Verification items for the finished model (mm, model axes). Coordinates: 2 decimals unless noted, no trailing zeros. Order: outer loops, then holes, each group sorted by start corner. A loop starts at its lowest first (then second) coordinate and runs counter-clockwise, first axis right, second up. Notation, with made-up numbers: M -19,-11.5 L 16,-11.5 A15 cw 16,6.5 Z; hole C -12.5,75 d9. An arc over 180 degrees is marked long. Return JSON: item names as keys, results as strings.
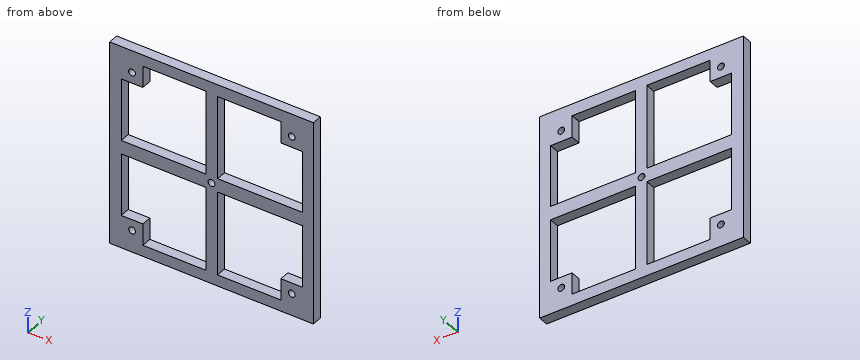
```python
from build123d import *

# Parameters (mm, degrees)
F0_W     = 59.944
F0_H     = 59.944
F0_W_2   = 25
F0_H_2   = 2
F0_W_3   = 6.35
F0_H_3   = 6.35
F1_DEPTH = 3
F2_D     = 2


# Not quite as in the source:
# - a feature names something its author has since deleted; it is built from what else it names


with BuildPart() as f1:
    # F0 (on Front) → F1 (new body)
    with BuildSketch(Plane.XZ):
        Rectangle(F0_W, F0_H)
        Polygon((-26.5568002729, 26.67), (-20.2068002729, 26.67), (-1.5568002729, 26.67), (-1.5568002729, 20.32), (-1.5568002729, 2), (-1.5568002729, 0), (-1.5568002729, -2), (-1.5568002729, -20.32), (-1.5568002729, -26.67), (-20.2068002729, -26.67), (-26.5568002729, -26.67), (-26.5568002729, -20.32), (-26.5568002729, -2), (-26.5568002729, 0), (-26.5568002729, 2), (-26.5568002729, 20.32), align=None, mode=Mode.SUBTRACT)
        Polygon((20.4331997271, 26.4424991059), (26.7831997271, 26.4424991059), (26.7831997271, 20.0924991059), (26.7831997271, 2), (26.7831997271, 0), (26.7831997271, -2), (26.7831997271, -20.32), (26.7831997271, -26.67), (20.4331997271, -26.67), (1.7831997271, -26.67), (1.7831997271, -20.32), (1.7831997271, -2), (1.7831997271, 0), (1.7831997271, 2), (1.7831997271, 20.0924991059), (1.7831997271, 26.4424991059), align=None, mode=Mode.SUBTRACT)
        with Locations((14.2831997271, 1)):
            Rectangle(F0_W_2, F0_H_2)
        with Locations((14.2831997271, -1)):
            Rectangle(F0_W_2, F0_H_2)
        with Locations((-14.0568002729, 1)):
            Rectangle(F0_W_2, F0_H_2)
        with Locations((-14.0568002729, -1)):
            Rectangle(F0_W_2, F0_H_2)
        Polygon((-20.2068002729, 26.4424991059), (-20.2068002729, 26.67), (-26.5568002729, 26.67), (-26.5568002729, 20.32), (-20.2068002729, 20.32), align=None)
        Polygon((26.7831997271, 20.0924991059), (26.7831997271, 26.4424991059), (20.4331997271, 26.4424991059), (20.4331997271, 20.32), (20.4331997271, 20.0924991059), align=None)
        with Locations((23.6081997271, -23.495)):
            Rectangle(F0_W_3, F0_H_3)
        with Locations((-23.3818002729, -23.495)):
            Rectangle(F0_W_3, F0_H_3)
    extrude(amount=F1_DEPTH)

    # F2 (through all)
    with Locations(Plane(origin=(0, 0, 0), x_dir=(1, 0, 0), z_dir=(0, 1, 0))):
        with Locations((23.6081997271, -23.2674991059), (0, 0), (23.6081997271, 23.495), (-23.3818002729, -23.495), (-23.3818002729, 23.495)):
            Hole(F2_D / 2)


solid = f1.part
```
Q1. Cross-section at B-B, the plane x = 0. Record the boundary of the cut face in (y, z).
Values:
{"outline": "M -3,-29.97 L 0,-29.97 L 0,-1 L -3,-1 Z; M -3,1 L 0,1 L 0,29.97 L -3,29.97 Z"}
Q2. Cross-section at C-C, the plane x = 15.5. Record the boundary of the cut face in (y, z).
Values:
{"outline": "M -3,-29.97 L 0,-29.97 L 0,-26.67 L -3,-26.67 Z; M -3,-2 L 0,-2 L 0,2 L -3,2 Z; M -3,26.44 L 0,26.44 L 0,29.97 L -3,29.97 Z"}
Q3. Cross-section at D-D, the plane z = -21.5. Record the boundary of the cut face in (x, y), and give its area (3 significant figures).
Values:
{"outline": "M -29.97,-3 L -20.21,-3 L -20.21,0 L -29.97,0 Z; M -1.56,-3 L 1.78,-3 L 1.78,0 L -1.56,0 Z; M 20.43,-3 L 29.97,-3 L 29.97,0 L 20.43,0 Z", "area": "67.9 mm^2"}
Q4. Cross-section at A-A, the plane z = 0. Record the boundary of the cut face in (x, y).
Values:
{"outline": "M -29.97,-3 L -1,-3 L -1,0 L -29.97,0 Z; M 1,-3 L 29.97,-3 L 29.97,0 L 1,0 Z"}
Q5. Material ranges on line 1 along Z through (x, y) = (-16, -2); line 2 along X through (y, z) = (-2.45, -16.5); line 3 along X through (y, z) = (-1.9, -25), recorded low to high.
Values:
{"line 1": "-29.97 to -26.67, -2 to 2, 26.67 to 29.97", "line 2": "-29.97 to -26.56, -1.56 to 1.78, 26.78 to 29.97", "line 3": "-29.97 to -20.21, -1.56 to 1.78, 20.43 to 29.97"}
